```python
from build123d import *

# Parameters (mm, degrees)
SKETCH2_W           = 78
SKETCH2_H           = 21
SKETCH2_W_2         = 10
SKETCH2_H_2         = 10
BOSS_EXTRUDE1_DEPTH = 50
CHAMFER1_SIZE       = 2.5
CHAMFER2_SIZE       = 0.5
SKETCH3_R           = 4.5
BOSS_EXTRUDE2_DEPTH = 25
BOSS_EXTRUDE3_START = 5
SKETCH4_R           = 95
SKETCH4_R_2         = 4.5
BOSS_EXTRUDE3_DEPTH = 18
SKETCH5_W           = 86
SKETCH5_H           = 12
CUT_EXTRUDE1_DEPTH  = 0.5
CIRPATTERN1_COUNT   = 4


with BuildPart() as part:
    # Sketch2 → Boss-Extrude1 (new body)
    with BuildSketch(Plane.XY):
        Rectangle(SKETCH2_W, SKETCH2_H)
        with Locations((-31, 4)):
            Rectangle(SKETCH2_W_2, SKETCH2_H_2, mode=Mode.SUBTRACT)
        with Locations((31, 4)):
            Rectangle(SKETCH2_W_2, SKETCH2_H_2, mode=Mode.SUBTRACT)
    extrude(amount=BOSS_EXTRUDE1_DEPTH)

    # Chamfer1
    chamfer1_edges = [part.edges().sort_by_distance(p)[0] for p in [
        (39, -10.5, 25),
        (-39, -10.5, 25),
    ]]
    chamfer(chamfer1_edges, length=CHAMFER1_SIZE)

    # Chamfer2
    chamfer2_edges = [part.edges().sort_by_distance(p)[0] for p in [
        (-39, 10.5, 25),
        (39, 10.5, 25),
    ]]
    chamfer(chamfer2_edges, length=CHAMFER2_SIZE)

    # Sketch3 → Boss-Extrude2 (add)
    with BuildSketch(Plane(origin=(0, 10.5, 0), x_dir=(1, 0, 0), z_dir=(0, 1, 0))):
        with Locations((0, -25)):
            Circle(SKETCH3_R)
    extrude(amount=BOSS_EXTRUDE2_DEPTH)

    # Sketch4 → Boss-Extrude3 (add)
    with BuildSketch(Plane(origin=(0, 10.5, 0), x_dir=(1, 0, 0), z_dir=(0, 1, 0)).offset(BOSS_EXTRUDE3_START)):
        with Locations((0, -25)):
            Circle(SKETCH4_R)
        with Locations((0, -25)):
            Circle(SKETCH4_R_2, mode=Mode.SUBTRACT)
    extrude(amount=BOSS_EXTRUDE3_DEPTH)

    # Sketch5 → Cut-Revolve1 (revolve, cut)
    with BuildSketch(Plane(origin=(0, 0, 0), x_dir=(0, 0, -1), z_dir=(1, 0, 0))):
        with Locations((27, 24.5)):
            Rectangle(SKETCH5_W, SKETCH5_H)
    revolve(axis=Axis((0, 10.5, 25), (0, 1, 0)), mode=Mode.SUBTRACT)

    # Sketch6 → Cut-Extrude1 (cut)
    with BuildSketch(Plane(origin=(0, 33.5, 0), x_dir=(1, 0, 0), z_dir=(0, 1, 0))):
        with BuildLine():
            Line((9, 58.006582115), (9, -16))
            Line((9, -16), (83.006582115, -16))
            ThreePointArc((83.006582115, -16), (59.03851571, 34.03851571), (9, 58.006582115))
        make_face()
    cut_extrude1 = extrude(amount=-CUT_EXTRUDE1_DEPTH, mode=Mode.SUBTRACT)

    # CirPattern1: Cut-Extrude1 ×4 about axis
    cirpattern1_axis = Axis((0, 0, 25), (0, 1, 0))
    for i in range(1, CIRPATTERN1_COUNT):
        add(cut_extrude1.rotate(cirpattern1_axis, i * 360 / CIRPATTERN1_COUNT), mode=Mode.SUBTRACT)


solid = part.part
```
Work out the finished part from the listing and answer in its coordinate system (mm). A direction names the side the tool comes from. Coordinates: 2 decimals unless noted, no trailing zeros. Write each loop counter-clockwise with the first axis right and the second up, starting at its lowest first coordinate (ties: lowest second). Pieces come first, ordered by that corner, then holes.
Q1. Each of these flat-tipped pins is pushed along its axis until it touches: pin 1 Ø1.5 at (x, z) = (-0.5, -42.5) entering from +Y; pin 2 Ø2 at (y, z) = (5, 39) entering from -X; pin 3 Ø6 at (x, y) = (13.5, 26) entering from +Z (1 decimal); pin 4 Ø12 at (x, y) = (-18, 1.5) entering from -Z. Where does it stop, or does it pass through?
Q2. Find the intervals of material crossed by line 1 (X direction, y = 2.5, z = 17); line 2 (X direction, y = 22, z = 24.5); line 3 (Y direction, x = 37.5, z = 30), in increasing order.
Q3. A cutting plane is placed at D-D, the plane x = -15.5. Give the vertices of the cut face in (y, z), then the cut area to 3 significant figures.
Q4. Which of the six approach directions +Z, -Z, +X, -X, +Y, -Y give full straight-line access (tool end or side, diameter ignored) to faces 4 (the face through (0, 35.5, 25)), 5 (the face through (2.419, 34.486, 21.206)), 6 (the face through (31, 9, 25))?
Q5. A cutting plane is placed at B-B, the plane z = 70. Give the vertices of the cut face in (x, y).
Q6. Determine the mould class of faces 1 (the face through (-59.596, 33.254, 83.476)), 2 (the face through (-36, 4, 25)), 3 (the face through (-2.703, 24.584, 16.416)) for opening direction Z: released by +Z, released by -Z, zero draft, split by the parting line, or undercut.
Q7. A cutting plane is placed at A-A, the plane y = 4.5. Give the vertices of the cut face in (x, z).
Q8. A cutting plane is placed at C-C, the plane x = -75. Give the vertices of the cut face in (y, z), then the cut area to 3 significant figures.
Findings below:
1. pin 1: stops at y = 33.5
1. pin 2: stops at x = -39
1. pin 3: passes through
1. pin 4: stops at z = 0
2. line 1: x = -39 to -36, -26 to 26, 36 to 39
2. line 2: x = -8.99 to 8.99
2. line 3: y = -9.5 to 10.5, 15.5 to 18.5, 30.5 to 33.5
3. outline: (-10.5, 0) - (10.5, 0) - (10.5, 50) - (-10.5, 50) - close; (15.5, -68.73) - (18.5, -68.73) - (18.5, 118.73) - (15.5, 118.73) - close; (30.5, -68.73) - (33.5, -68.73) - (33.5, -57.04) - (33, -57.04) - (33, 16) - (33.5, 16) - (33.5, 34) - (33, 34) - (33, 107.04) - (33.5, 107.04) - (33.5, 118.73) - (30.5, 118.73) - close
3. area: 2,100 mm2
4. face 4: +Z, -Z, +X, -X, +Y
4. face 5: +Y
4. face 6: +Z, -Z
5. outline: (-83.67, 15.5) - (83.67, 15.5) - (83.67, 18.5) - (-83.67, 18.5) - close; (-83.67, 30.5) - (83.67, 30.5) - (83.67, 33.5) - (70.33, 33.5) - (70.33, 33) - (9, 33) - (9, 33.5) - (-9, 33.5) - (-9, 33) - (-70.33, 33) - (-70.33, 33.5) - (-83.67, 33.5) - close
6. face 1: undercut
6. face 2: zero draft
6. face 3: split by the parting line
7. outline: (-39, 0) - (-36, 0) - (-36, 50) - (-39, 50) - close; (-26, 0) - (26, 0) - (26, 50) - (-26, 50) - close; (36, 0) - (39, 0) - (39, 50) - (36, 50) - close
8. outline: (15.5, -33.31) - (18.5, -33.31) - (18.5, 83.31) - (15.5, 83.31) - close; (30.5, -33.31) - (33.5, -33.31) - (33.5, -11.69) - (33, -11.69) - (33, 16) - (33.5, 16) - (33.5, 34) - (33, 34) - (33, 61.69) - (33.5, 61.69) - (33.5, 83.31) - (30.5, 83.31) - close
8. area: 672 mm2
